Geometry: final body of the model. Coordinates: model frame, mm. Face numbers are marked on the shaded views. A direction names the side the tool comes from. Give positions to 0.01 mm unless a question says otherwise; leave off trailing zeros.
Q1. Section A-A (z = 25). State how many separate pieces and enclosed holes the cut face has, plus the area to 3 significant figures.
Q2. Pin query (flat end, axial travel): pin 1 Ø1.5 at (x, z) = (-21, 8) entering from -Y; pin 2 Ø4.5 at (y, z) = (87.5, 34.5) entering from +X; pin 3 Ø3.5 at (x, z) = (-23.5, 10.25) entering from -Y; pin 4 Ø4 at (x, y) = (-11, -45) entering from +Z. Return the tip coordinate at first contact, or that it passes through.
Q3. Reachability of the marked faces 1 and 2 from +Z, -Z, +X, -X, +Y, -Y: full face, straight path, thin tool, end or side. Return the list, or none.
Q4. Line query: line 1 (X direction, y = -72, z = 21.5); line 2 (Y direction, x = 40.5, z = 16); line 3 (Z direction, x = -22.5, y = -65). Output: solid intervals per line, ascending.
from build123d import *

# Parameters (mm, degrees)
SKETCH_W             = 118
SKETCH_H             = 179
PAD_DEPTH            = 63
PAD_DEPTH_BACK       = 2
SKETCH001_W          = 110
SKETCH001_H          = 175
POCKET_DEPTH         = 63.001
FILLET_R             = 2
FILLET001_R          = 6
CHAMFER_SIZE         = 3.999
POCKET001_DEPTH      = 83.5
POCKET001_DEPTH_BACK = -1000
POCKET002_DEPTH      = 63.001
CHAMFER001_SIZE      = 1.999
POCKET003_DEPTH      = 2.001
POCKET003_DEPTH_BACK = -63.001
SKETCH006_W          = 2
SKETCH006_H          = 2
POCKET004_DEPTH      = 5
SKETCH007_R          = 2
POCKET005_DEPTH      = 89.501


with BuildPart() as part:
    # Sketch → Pad (new body, two sides)
    with BuildSketch(Plane.XY) as pad_sk:
        Rectangle(SKETCH_W, SKETCH_H)
    extrude(amount=PAD_DEPTH)
    extrude(pad_sk.sketch, amount=-PAD_DEPTH_BACK)

    # Sketch001 → Pocket (cut, through all)
    with BuildSketch(Plane.XY):
        with Locations((0, -2)):
            Rectangle(SKETCH001_W, SKETCH001_H)
    extrude(amount=POCKET_DEPTH, mode=Mode.SUBTRACT)

    # Fillet
    fillet_edges = [part.edges().sort_by_distance(p)[0] for p in [
        (55, 85.5, 31.5),
        (-55, 85.5, 31.5),
    ]]
    fillet(fillet_edges, radius=FILLET_R)

    # Fillet001
    fillet001_edges = [part.edges().sort_by_distance(p)[0] for p in [
        (-59, 89.5, 30.5),
        (59, 89.5, 30.5),
    ]]
    fillet(fillet001_edges, radius=FILLET001_R)

    # Chamfer
    chamfer_edges = [part.edges().sort_by_distance(p)[0] for p in [
        (-55, -3, 63),
    ]]
    chamfer(chamfer_edges, length=CHAMFER_SIZE)

    # Sketch003 → Pocket001 (cut, two sides)
    with BuildSketch(Plane.XZ) as pocket001_sk:
        Polygon((-55, 59), (-57, 57), (-55, 55), (55, 55), (57, 57), (55, 59), align=None)
    extrude(amount=-POCKET001_DEPTH, mode=Mode.SUBTRACT)
    extrude(pocket001_sk.sketch, amount=-POCKET001_DEPTH_BACK, mode=Mode.SUBTRACT)

    # Sketch004 → Pocket002 (cut, through all)
    with BuildSketch(Plane.XY):
        Polygon((-59, -70.5), (-59, 70.5), (-57, 68.5), (-55, 70.5), (-55, -70.5), (-57, -68.5), align=None)
    extrude(amount=POCKET002_DEPTH, mode=Mode.SUBTRACT)

    # Chamfer001
    chamfer001_edges = [part.edges().sort_by_distance(p)[0] for p in [
        (0, -89.5, -2),
    ]]
    chamfer(chamfer001_edges, length=CHAMFER001_SIZE)

    # Sketch005 → Pocket003 (cut, two sides)
    with BuildSketch(Plane.XY) as pocket003_sk:
        Polygon((-58.5, -89.5), (-58, -87.5), (-56, -87.5), (-56.5, -89.5), align=None)
        Polygon((58.5, -89.5), (56.5, -89.5), (56, -87.5), (58, -87.5), align=None)
    extrude(amount=-POCKET003_DEPTH, mode=Mode.SUBTRACT)
    extrude(pocket003_sk.sketch, amount=-POCKET003_DEPTH_BACK, mode=Mode.SUBTRACT)

    # Sketch006 (on DatumPlane) → Pocket004 (cut)
    with BuildSketch(Plane.XY.offset(57)):
        with Locations((-56, -88.5)):
            Rectangle(SKETCH006_W, SKETCH006_H)
        with Locations((56, -88.5)):
            Rectangle(SKETCH006_W, SKETCH006_H)
    extrude(amount=POCKET004_DEPTH, mode=Mode.SUBTRACT)

    # Sketch007 → Pocket005 (cut, through all)
    with BuildSketch(Plane.XZ):
        with Locations((-23.5, 10.25)):
            Circle(SKETCH007_R)
        with Locations((-23.5, 49.75)):
            Circle(SKETCH007_R)
        Polygon((0, 43.5), (-47, 43.5), (-47, 30), (-47, 16.5), (0, 16.5), (0, 30), align=None)
    extrude(amount=-POCKET005_DEPTH, mode=Mode.SUBTRACT)


solid = part.part
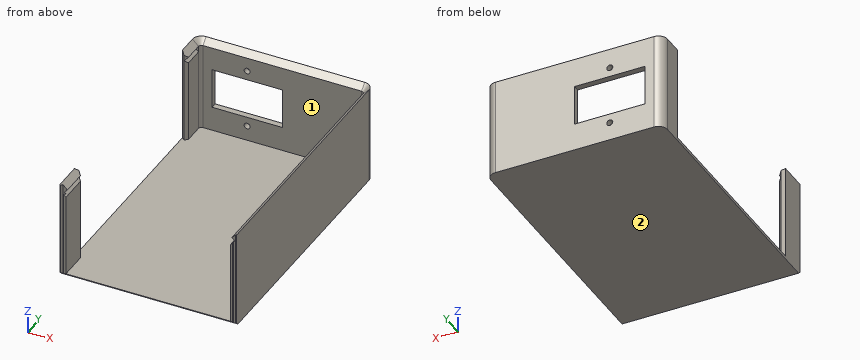
Computed:
1. separate pieces: 3
1. enclosed holes: 0
1. area: 1,110 mm2
2. pin 1: stops at y = 85.5
2. pin 2: stops at x = 58.74
2. pin 3: passes through
2. pin 4: stops at z = 0
3. face 1: +Z, -Y
3. face 2: -Z, +X, -X, +Y, -Y
4. line 1: x = -59 to -55, 55 to 59
4. line 2: y = 85.5 to 89.5
4. line 3: z = -2 to 0
